Could you check a few things on this model? Use its own coordinates, in mm. Face numbers are marked on the shaded views. A direction names the side the tool comes from. Round coordinates to 2 decimals unless told otherwise and drop trailing zeros. Write each loop counter-clockwise with the first axis right and the second up, starting at its lowest first coordinate (ties: lowest second). Pieces come first, ordered by that corner, then holes. Notation, with made-up numbers: (29, 22) -> (44, 22) arc R17 cw to (44, 48) -> close; hole circle Ø3 at (85.5, 1). An arc over 180 degrees is marked (long way). Answer in a Markdown table with one row per item.
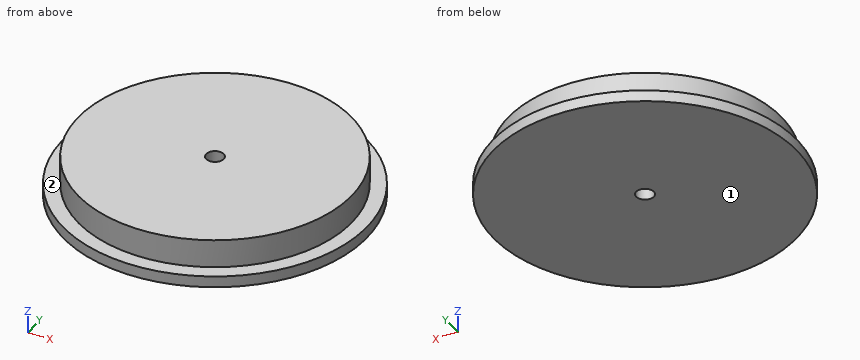
Autodesk Fusion 360 part; units mm, degrees
sketch "Flange" plane through (0, 0, 0) normal (0, 0, 1) x (1, 0, 0)
  circle A0 centre (0, 0) radius 21.5
extrude "Flange (1)" add sketch "Flange" along normal blind 1.6
ref_plane "WorkPlane1" through (0, 0, 1.6) normal (0, 0, 1) x (1, 0, 0)
sketch "Press-fit body" plane through (0, 0, 1.6) normal (0, 0, 1) x (1, 0, 0)
  circle A0 centre (0, 0) radius 19.35
extrude "Press-fit body (1)" add sketch "Press-fit body" along normal blind 4
sketch "Puller pilot" plane through (0, 0, 0) normal (0, 0, 1) x (1, 0, 0)
  circle A0 centre (0, 0) radius 1.25
extrude "Puller pilot (1)" cut sketch "Puller pilot" along normal mid plane 11.2
1) For pin 1 (2 mm diameter, centred on x = -6.5, y = -10.5, fed in from -Z); pin 2 (1.5 mm diameter, centred on x = -3.5, z = 1, fed in from -Y); pin 3 (2 mm diameter, centred on x = 0, y = 0, fed in from -Z); pin 4 (1.5 mm diameter, centred on y = 4, z = 3.5, fed in from +X), each with a flat end and sliding along its axis, tell me the tip position at first contact or that it passes through.
Findings:
| item | result |
|---|---|
| pin 1 | stops at z = 0 |
| pin 2 | stops at y = -21.32 |
| pin 3 | passes through |
| pin 4 | stops at x = 19.08 |
2) For the marked faces 1 and 2, which set-ups out of +Z, -Z, +X, -X, +Y, -Y let a thin tool reach every point of the face, with its end or its side?
Findings:
| item | result |
|---|---|
| face 1 | -Z, +X, -X, +Y, -Y |
| face 2 | +Z |
3) Imagine slicing it at D-D, the plane x = -5.5. Please give me the cut outline in (y, z), plus the area to 3 significant figures.
Findings:
| item | result |
|---|---|
| outline | (-20.78, 0) -> (20.78, 0) -> (20.78, 1.6) -> (18.55, 1.6) -> (18.55, 5.6) -> (-18.55, 5.6) -> (-18.55, 1.6) -> (-20.78, 1.6) -> close |
| area | 215 mm^2 |
4) Please list where these lines run through material, in increasing order: line 1 (Y direction, x = 0, z = 2.35); line 2 (Z direction, x = 12, y = 16); line 3 (X direction, y = -14, z = 3.6).
Findings:
| item | result |
|---|---|
| line 1 | y = -19.35 to -1.25, 1.25 to 19.35 |
| line 2 | z = 0 to 1.6 |
| line 3 | x = -13.36 to 13.36 |
5) Imagine slicing it at C-C, the plane z = 3.85. Please give me the cut outline in (x, y).
Findings:
| item | result |
|---|---|
| outline | circle Ø38.7 at (0, 0); hole circle Ø2.5 at (0, 0) |
6) Imagine slicing it at A-A, the plane x = 0. Please give me the cut outline in (y, z), plus the area to 3 significant figures.
Findings:
| item | result |
|---|---|
| outline | (-21.5, 0) -> (-1.25, 0) -> (-1.25, 5.6) -> (-19.35, 5.6) -> (-19.35, 1.6) -> (-21.5, 1.6) -> close; (1.25, 0) -> (21.5, 0) -> (21.5, 1.6) -> (19.35, 1.6) -> (19.35, 5.6) -> (1.25, 5.6) -> close |
| area | 210 mm^2 |
